Read the model definition and answer for the solid it produces. Units are mm, in the model's axes. Coordinates: 2 decimals unless noted, no trailing zeros. Loops run counter-clockwise (first coordinate to the right, second up) from the corner with the lowest first, then second, coordinate; pieces in that order, holes last. Notation, with made-up numbers: (40, 53.5) -> (57, 53.5) arc R20 cw to (57, 76.5) -> close; hole circle Ø3 at (85.25, 56). An arc over 180 degrees is marked (long way). Answer in a Markdown table with one row per item.
Autodesk Inventor part; units mm, degrees
ref_plane "YZ Plane" through (0, 0, 0) normal (1, 0, 0) x (0, 1, 0)
ref_plane "XZ Plane" through (0, 0, 0) normal (0, 1, 0) x (-1, 0, 0)
ref_plane "XY Plane" through (0, 0, 0) normal (0, 0, 1) x (1, 0, 0)
sketch "Sketch1" plane through (0, 0, 0) normal (0, 0, 1) x (1, 0, 0)
  line L0 (120.396, 63.5) -> (-114.3, 63.5)
  line L1 (-114.3, 63.5) -> (-114.3, -63.5)
  line L2 (-114.3, -63.5) -> (120.396, -63.5)
  line L3 (120.396, -63.5) -> (120.396, 63.5)
  point P0 (0, 0)
  dimension "d0" = 234.696
  dimension "d1" = 127
extrude "Plate1" add sketch "Sketch1" along normal blind 3.048
sketch "Sketch2" plane through (0, 0, 3.048) normal (0, 0, 1) x (1, 0, 0)
  line L0 (-114.3, 63.5) -> (-114.3, -63.5)
  line L1 (-114.3, -63.5) -> (-114.3, -60.325)
  line L2 (-114.3, -60.325) -> (-73.152, -60.325)
  line L3 (-73.152, -60.325) -> (-35.052, -60.325)
  line L4 (-35.052, -60.325) -> (3.048, -60.325)
  line L5 (3.048, -60.325) -> (41.148, -60.325)
  line L6 (41.148, -60.325) -> (79.248, -60.325)
  line L7 (79.248, -60.325) -> (120.396, -60.325)
  line L8 (120.396, -63.5) -> (120.396, 63.5)
  point P0 (0, 0)
  dimension "d3" = 3.175
  dimension "d4" = 41.148
  dimension "d5" = 38.1
  dimension "d6" = 38.1
  dimension "d7" = 38.1
  dimension "d8" = 38.1
hole "Hole1" at (-73.152, -60.325, 3.048) at (-35.052, -60.325, 3.048) at (3.048, -60.325, 3.048) at (41.148, -60.325, 3.048) at (79.248, -60.325, 3.048) direction (0, 0, -1) diameter 4.4958 depth 3.048
sketch "Sketch3" plane through (0, 0, 3.048) normal (0, 0, 1) x (1, 0, 0)
  line L0 (-114.3, -63.5) -> (120.396, -63.5)
  line L1 (-114.3, -63.5) -> (-114.3, -50.8)
  line L2 (-114.3, 63.5) -> (-114.3, -63.5)
  line L3 (-114.3, -50.8) -> (-114.3, -25.4)
  line L4 (-114.3, -25.4) -> (-88.9, -25.4)
  line L5 (-88.9, -25.4) -> (-88.9, 31.6)
  line L6 (-88.9, 31.6) -> (-43.9, 31.6)
  line L7 (-43.9, 31.6) -> (-43.9, -25.4)
  line L8 (-43.9, -25.4) -> (-88.9, -25.4)
  line L9 (-43.9, 31.6) -> (-36.28, 31.6)
  line L10 (-36.28, 31.6) -> (-36.28, -25.4)
  line L11 (-36.28, -25.4) -> (8.72, -25.4)
  line L12 (8.72, -25.4) -> (8.72, 31.6)
  line L13 (8.72, 31.6) -> (-36.28, 31.6)
  point P0 (0, 0)
  dimension "d16" = 12.7
  dimension "d17" = 25.4
  dimension "d18" = 25.4
  dimension "d19" = 57
  dimension "d20" = 45
  dimension "d21" = 7.62
  dimension "d22" = 45
sketch "Sketch4" plane through (0, 0, 3.048) normal (0, 0, 1) x (1, 0, 0)
  line L0 (-88.9, 31.6) -> (-43.9, 31.6)
  line L1 (-43.9, -25.4) -> (-88.9, -25.4)
  line L2 (-36.28, -25.4) -> (8.72, -25.4)
  line L3 (8.72, 31.6) -> (-36.28, 31.6)
  line L4 (-66.4, 31.6) -> (-66.4, 26.6)
  line L5 (-66.4, -25.4) -> (-66.4, -20.4)
  line L6 (-13.78, -25.4) -> (-13.78, -20.4)
  line L7 (-13.78, 31.6) -> (-13.78, 26.6)
  point P0 (0, 0)
  dimension "d23" = 5
  dimension "d24" = 5
  dimension "d25" = 5
  dimension "d26" = 5
hole "Hole2" at (-66.4, 26.6, 3.048) at (-66.4, -20.4, 3.048) at (-13.78, -20.4, 3.048) at (-13.78, 26.6, 3.048) direction (0, 0, -1) diameter 4.4958 depth 3.048
sketch "Sketch5" plane through (0, 0, 3.048) normal (0, 0, 1) x (1, 0, 0)
  line L0 (-114.3, -63.5) -> (120.396, -63.5)
  line L1 (120.396, -63.5) -> (120.396, -50.8)
  line L2 (120.396, -63.5) -> (120.396, 63.5)
  line L3 (120.396, -50.8) -> (120.396, 0)
  line L4 (120.396, 0) -> (94.996, 0)
  line L5 (94.996, 0) -> (94.996, 61.6)
  line L6 (94.996, 61.6) -> (71.996, 61.6)
  line L7 (8.72, -25.4) -> (8.72, 31.6)
  line L8 (94.996, 0) -> (33.396, 0)
  line L9 (33.396, 0) -> (33.396, 23)
  line L10 (94.996, 0) -> (94.996, 23)
  point P0 (0, 0)
  dimension "d34" = 12.7
  dimension "d35" = 50.8
  dimension "d36" = 25.4
  dimension "d37" = 61.6
  dimension "d38" = 23
  dimension "d46" = 61.6
  dimension "d47" = 23
hole "Hole3" at (33.396, 23, 3.048) at (94.996, 0, 3.048) direction (0, 0, -1) diameter 3.2766 depth 3.048
sketch "Sketch6" plane through (0, 0, 3.048) normal (0, 0, 1) x (1, 0, 0)
  line L0 (-114.3, -63.5) -> (-114.3, 63.5)
  line L1 (-114.3, 63.5) -> (-114.3, 50.8)
  line L2 (-114.3, 50.8) -> (-38.1, 50.8)
  line L3 (-38.1, 50.8) -> (38.1, 50.8)
  point P0 (0, 0)
  dimension "d48" = 12.7
  dimension "d49" = 76.2
  dimension "d50" = 76.2
hole "Hole4" at (-38.1, 50.8, 3.048) at (38.1, 50.8, 3.048) direction (0, 0, -1) diameter 3.2766 end through all
sketch "Sketch7" plane through (0, 0, 3.048) normal (0, 0, 1) x (1, 0, 0)
  line L0 (120.396, -63.5) -> (69.596, -63.5)
  line L1 (120.396, -63.5) -> (-114.3, -63.5)
  line L2 (69.596, -63.5) -> (69.596, -38.1)
  line L3 (69.596, -38.1) -> (44.196, -38.1)
  line L4 (44.196, -38.1) -> (18.796, -38.1)
  point P0 (0, 0)
  dimension "d58" = 50.8
  dimension "d59" = 25.4
  dimension "d60" = 25.4
  dimension "d61" = 25.4
hole "Hole5" at (69.596, -38.1, 3.048) direction (0, 0, -1) diameter 6.7564 depth 3.048
equation "\"d14\" = Thickness"
equation "\"d32\" = Thickness"
equation "\"d44\" = Thickness"
equation "\"d56\" = Thickness"
equation "\"d67\" = Thickness"
equation "\"d2\" = Thickness"
equation "\"BendRadius\" = Thickness"
equation "\"BendReliefWidth\" = Thickness"
equation "\"BendReliefDepth\" = 0.5 * Thickness"
equation "\"CornerReliefSize\" = 4 * Thickness"
equation "\"MinimumRemnant\" = 2 * Thickness"
equation "\"TransitionRadius\" = BendRadius"
equation "\"JacobiRadiusSize\" = BendRadius"
equation "\"GapSize\" = Thickness"
properties part number "sheetmetalback2.0"
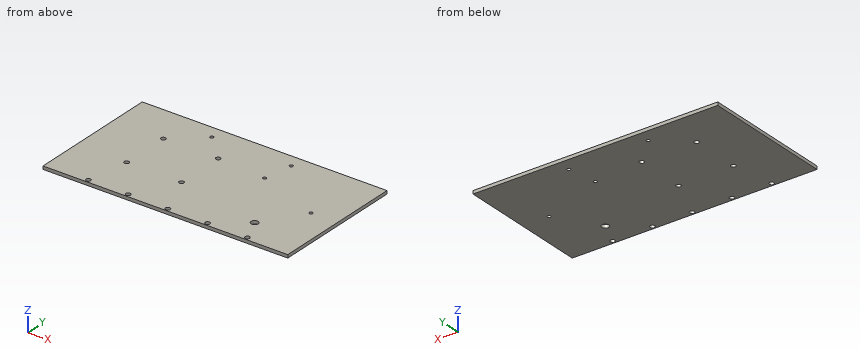
1. Find the intervals of material crossed by probe 1 along X at (y, z) = (26.6, 1); probe 2 along Y at (x, z) = (-66.4, 1.55); probe 3 along X at (y, z) = (23, 0.9), in increasing order.
A:
| item | result |
|---|---|
| probe 1 | x = -114.3 to -68.65, -64.15 to -16.03, -11.53 to 120.4 |
| probe 2 | y = -63.5 to -22.65, -18.15 to 24.35, 28.85 to 63.5 |
| probe 3 | x = -114.3 to 31.76, 35.03 to 120.4 |
2. Given pin 1 Ø1 at (x, y) = (1.5, -33.5) entering from -Z, flat-ended and moving along its own axis, determine where the tip first touches the part or whether it passes through.
A:
| item | result |
|---|---|
| pin 1 | stops at z = 0 |
3. A cutting plane is placed at A-A on x = -13.78. Give the vertices of the cut face in (y, z).
A:
| item | result |
|---|---|
| outline | (-63.5, 0) -> (-22.65, 0) -> (-22.65, 3.05) -> (-63.5, 3.05) -> close; (-18.15, 0) -> (24.35, 0) -> (24.35, 3.05) -> (-18.15, 3.05) -> close; (28.85, 0) -> (63.5, 0) -> (63.5, 3.05) -> (28.85, 3.05) -> close |
4. A cutting plane is placed at B-B on y = -20.4. Give the vertices of the cut face in (x, z), and give its area (3 significant figures).
A:
| item | result |
|---|---|
| outline | (-114.3, 0) -> (-68.65, 0) -> (-68.65, 3.05) -> (-114.3, 3.05) -> close; (-64.15, 0) -> (-16.03, 0) -> (-16.03, 3.05) -> (-64.15, 3.05) -> close; (-11.53, 0) -> (120.4, 0) -> (120.4, 3.05) -> (-11.53, 3.05) -> close |
| area | 688 mm2 |
